```python
from build123d import *

# Parameters (mm, degrees)
EXTRUDE010_DEPTH           = 14
EXTRUDE010_PLACEMENT_ANGLE = 90
BOX023_W                   = 17.5
BOX023_H                   = 14
BOX023_DEPTH               = 36


with BuildPart() as extrude010:
    # Sketch014 → Extrude010 (new body)
    with BuildSketch(Plane.XZ):
        with BuildLine():
            ThreePointArc((-4.8, 1.5), (-6.3, 0), (-4.8, -1.5))
            Line((-4.8, -1.5), (0, -1.5))
            ThreePointArc((0, -1.5), (1.5, 0), (0, 1.5))
            Line((-4.8, 1.5), (0, 1.5))
        make_face()
    extrude(amount=EXTRUDE010_DEPTH)


with BuildPart() as extrude010_1:
    # Extrude010 placement: moved
    add(extrude010.part.moved(Location((86.5, 27.25, -27))).rotate(Axis((86.5, 27.25, -27), (0, -1, 0)), EXTRUDE010_PLACEMENT_ANGLE))


with BuildPart() as cut005:
    # Box023 → Box023 (new body)
    with BuildSketch(Plane(origin=(72.25, 13.25, -36), x_dir=(1, 0, 0), z_dir=(0, 0, 1))):
        with Locations((8.75, 7)):
            Rectangle(BOX023_W, BOX023_H)
    extrude(amount=BOX023_DEPTH)

    # Cut005: cut Extrude010
    add(extrude010_1.part, mode=Mode.SUBTRACT)


with BuildPart() as cut005_1:
    # Cut005 placement: moved
    add(cut005.part.moved(Location((0, 3, 0))))


solid = cut005_1.part
```
Check sheet for the modelled part. Datum: model origin and axes. Units: mm. A direction names the side the tool comes from. Coordinates: 2 decimals unless noted, no trailing zeros. Write each loop counter-clockwise with the first axis right and the second up, starting at its lowest first coordinate (ties: lowest second). Pieces come first, ordered by that corner, then holes. Notation, with made-up numbers: M 23.5,-6 L 40.5,-6 A13 ccw 40.5,9 Z; hole C 46.25,-30 d8. An arc over 180 degrees is marked long. Use one line per item in the form item = value.
Item 1: Set-up check for faces 1 (the face through (81, 23, 0)), 2 (the face through (86.5, 23.3, -25.5)): record each of +Z, -Z, +X, -X, +Y, -Y from which the full face is reachable in a straight line by a thin tool's end or side.
Answer below:
face_1 = +Z, +X, -X, +Y, -Y
face_2 = +Y, -Y
Item 2: Release check for a two-part mould opening along X. For faces 3 (the face through (72.25, 23, -18)), 4 (the face through (81, 16.25, -18)), 5 (the face through (88, 23, -29)) record: pulls with the +X half, pulls with the -X half, needs draft (parallel to the pull), parting line crosses it, or undercut.
Answer below:
face_3 = pulls with the -X half
face_4 = needs draft
face_5 = undercut
Item 3: Sectioned sample at A-A, the plane x = 86.5. Record the cut outline in (y, z), and give its area (3 significant figures).
Answer below:
outline = M 16.25,-36 L 30.25,-36 L 30.25,-33.3 L 16.25,-33.3 Z; M 16.25,-25.5 L 30.25,-25.5 L 30.25,0 L 16.25,0 Z
area = 395 mm^2
Item 4: Sectioned sample at B-B, the plane y = 20.5. Record the cut outline in (x, z), and give its area (3 significant figures).
Answer below:
outline = M 72.25,-36 L 89.75,-36 L 89.75,0 L 72.25,0 Z; hole M 85,-31.8 A1.5 ccw 88,-31.8 L 88,-27 A1.5 ccw 85,-27 Z
area = 609 mm^2
Item 5: Material ranges on L1, parallel to X at y = 26, z = -28.5; L2, parallel to X at y = 27.25, z = -26; L3, parallel to Z at x = 86, y = 29, recorded low to high. Write a range as from..to.
Answer below:
L1 = 72.25..85, 88..89.75
L2 = 72.25..85.38, 87.62..89.75
L3 = -36..-33.21, -25.59..0
